```python
from build123d import *

# Parameters (mm, degrees)
SKETCH1_R           = 10
SKETCH1_R_2         = 8.657914019
BOSS_EXTRUDE1_DEPTH = 10
BOSS_EXTRUDE2_START = -4
SKETCH1_3_R         = 13
SKETCH1_3_R_2       = 10
SKETCH1_3_R_3       = 8.657914019
BOSS_EXTRUDE2_DEPTH = 4
CHAMFER1_SIZE       = 2
FILLET1_R           = 0.4
FILLET2_R           = 0.4
FILLET3_R           = 0.4


with BuildPart() as part:
    # Sketch1 → Boss-Extrude1 (new body)
    with BuildSketch(Plane.XY):
        Circle(SKETCH1_R)
        Circle(SKETCH1_R_2, mode=Mode.SUBTRACT)
    extrude(amount=BOSS_EXTRUDE1_DEPTH)

    # Sketch1_3 → Boss-Extrude2 (add)
    # profile 1 of 2: a face of its own
    with BuildSketch(Plane.XY.offset(BOSS_EXTRUDE2_START)):
        Circle(SKETCH1_3_R)
        Circle(SKETCH1_3_R_2, mode=Mode.SUBTRACT)
    # profile 2 of 2: a face of its own
    with BuildSketch(Plane.XY.offset(BOSS_EXTRUDE2_START)):
        Circle(SKETCH1_3_R_2)
        Circle(SKETCH1_3_R_3, mode=Mode.SUBTRACT)
    extrude(amount=BOSS_EXTRUDE2_DEPTH)

    # Chamfer1
    chamfer1_edges = [part.edges().sort_by_distance(p)[0] for p in [
        (-13, 0, -4),
    ]]
    chamfer(chamfer1_edges, length=CHAMFER1_SIZE)

    # Fillet1
    fillet1_edges = [part.edges().sort_by_distance(p)[0] for p in [
        (-8.657914019, 0, -4),
    ]]
    fillet(fillet1_edges, radius=FILLET1_R)

    # Fillet2
    fillet2_edges = [part.edges().sort_by_distance(p)[0] for p in [
        (-13, 0, -2),
        (-11, 0, -4),
    ]]
    fillet(fillet2_edges, radius=FILLET2_R)

    # Fillet3
    fillet3_edges = [part.edges().sort_by_distance(p)[0] for p in [
        (-13, 0, 0),
    ]]
    fillet(fillet3_edges, radius=FILLET3_R)


solid = part.part
```
For this review, take the finished solid that the model builds, in its own axes (mm). A direction names the side the tool comes from. Coordinates: 2 decimals unless noted, no trailing zeros. Loops run counter-clockwise (first coordinate to the right, second up) from the corner with the lowest first, then second, coordinate; pieces in that order, holes last. Notation, with made-up numbers: (84.25, 60) -> (115.25, 60) arc R30 ccw to (115.25, 82) -> close; hole circle Ø2 at (7, -1.75). An arc over 180 degrees is marked (long way). Return JSON: item names as keys, results as strings. Group by question number.
(1) For pin 1 Ø4 at (x, z) = (5.5, 5.5) entering from +Y; pin 2 Ø4 at (x, z) = (10.5, 7) entering from +Y; pin 3 Ø6 at (x, z) = (-8.5, 8) entering from +Y, all flat-tipped, find the tip position at first contact; note any pin that passes through.
(2) Consider section A-A, the plane z = 3.75. Give the boundary of the cut face in (x, y).
(3) Mouldability with a two-part tool opening along Y and no side actions: class faces 3 (the flat face through (0, 9, 10)), 4 (the cylindrical face through (-2.17, -9.76, 4.93)), 5 (the cylindrical face through (-6.38, 5.85, 3.1)) as pulls with the +Y half, pulls with the -Y half, needs draft (parallel to the pull), parting line crosses it, or undercut.
(4) To check wall thickness, follow L1, parallel to Y at x = 0, z = 1; L2, parallel to Y at x = 6, z = 9; L3, parallel to X at y = 2, z = 1.5. State the ranges of each line that lie inside material, in increasing order.
(5) Tool access review of faces 1 (the flat face through (-2, -9, -4)), 2 (the flat face through (-8, 7, 0)): name each direction out of +Z, -Z, +X, -X, +Y, -Y from which nothing blocks a thin tool from reaching the whole face with its end or side.
Results below:
{
 "1": {"pin 1": "stops at y = 9.37", "pin 2": "stops at y = 5.27", "pin 3": "stops at y = 8.35"},
 "2": {"outline": "circle Ø20 at (0, 0); hole circle Ø17.32 at (0, 0)"},
 "3": {"face 3": "needs draft", "face 4": "parting line crosses it", "face 5": "undercut"},
 "4": {"L1": "y = -10 to -8.66, 8.66 to 10", "L2": "y = -8 to -6.24, 6.24 to 8", "L3": "x = -9.8 to -8.42, 8.42 to 9.8"},
 "5": {"face 1": "-Z, +X, -X, +Y, -Y", "face 2": "+Z"}
}
